```python
from build123d import *

# Parameters (mm, degrees)
ESQUISSE1_W             = 148.59
ESQUISSE1_H             = 2.5
ESQUISSE1_H_2           = 20
BOSS_EXTRU_2_DEPTH      = 5
BOSS_EXTRU_4_DEPTH      = 0.001
BOSS_EXTRU_4_DEPTH_BACK = 2.5
ESQUISSE2_W             = 148.59
ESQUISSE2_H             = 43.5
ESQUISSE3_R             = 2
ENL_V_MAT_EXTRU_1_DEPTH = 5
BOSS_EXTRU_9_DEPTH      = 148
ENL_V_MAT_EXTRU_2_DEPTH = 148
ENL_V_MAT_EXTRU_3_DEPTH = 158
ESQUISSE7_W             = 74.295
ESQUISSE7_H             = 5.75
BOSS_EXTRU_10_DEPTH     = 11
ESQUISSE8_W             = 148
ESQUISSE8_H             = 6.4
BOSS_EXTRU_11_DEPTH     = 40


with BuildPart() as part:
    # Esquisse1 → Boss.-Extru.2 (new body)
    with BuildSketch(Plane(origin=(0, 0, 0), x_dir=(1, 0, 0), z_dir=(0, 1, 0))):
        with Locations((-5.161134174, 17.745562161)):
            Rectangle(ESQUISSE1_W, ESQUISSE1_H)
        with Locations((-5.161134174, 28.995562161)):
            Rectangle(ESQUISSE1_W, ESQUISSE1_H_2)
    extrude(amount=BOSS_EXTRU_2_DEPTH)

    # Esquisse2 → Boss.-Extru.4 (add, two sides: drawn at the far end of the back side and taken through both)
    with BuildSketch(Plane(origin=(0, 0, -38.995562161), x_dir=(-1, 0, 0), z_dir=(0, 0, -1)).offset(-BOSS_EXTRU_4_DEPTH_BACK)):
        with Locations((5.161134174, 26.75)):
            Rectangle(ESQUISSE2_W, ESQUISSE2_H)
    extrude(amount=BOSS_EXTRU_4_DEPTH + BOSS_EXTRU_4_DEPTH_BACK)

    # Esquisse3 → Enlèv. mat.-Extru.1 (cut)
    with BuildSketch(Plane.XZ):
        with Locations(Location((-69.456134174, -25.995562161, 0), (0, 0, 270))):
            Circle(ESQUISSE3_R)
        with Locations(Location((59.133865826, -25.995562161, 0), (0, 0, 270))):
            Circle(ESQUISSE3_R)
    extrude(amount=-ENL_V_MAT_EXTRU_1_DEPTH, mode=Mode.SUBTRACT)

    # Esquisse4 → Boss.-Extru.9 (add)
    with BuildSketch(Plane.ZY.offset(79.456134174)):
        Polygon((-38.996562161, 5), (-38.996562161, 48.5), (-53.996562161, 48.5), (-53.996562161, 20), align=None)
    extrude(amount=-BOSS_EXTRU_9_DEPTH)

    # Esquisse5 → Enlèv. mat.-Extru.2 (cut)
    with BuildSketch(Plane.XY.offset(-36.495562161)):
        with BuildLine():
            ThreePointArc((31.986365826, 33.75), (28.486365826, 30.25), (31.986365826, 26.75))
            Line((31.986365826, 26.75), (31.986365826, 33.75))
        make_face()
        with BuildLine():
            Line((31.986365826, 33.75), (31.986365826, 26.75))
            ThreePointArc((31.986365826, 26.75), (34.46123956, 27.775126266), (35.486365826, 30.25))
            ThreePointArc((35.486365826, 30.25), (34.46123956, 32.724873734), (31.986365826, 33.75))
        make_face()
        with BuildLine():
            ThreePointArc((-38.808634174, 30.25), (-39.83376044, 32.724873734), (-42.308634174, 33.75))
            Line((-42.308634174, 33.75), (-42.308634174, 26.75))
            ThreePointArc((-42.308634174, 26.75), (-39.83376044, 27.775126266), (-38.808634174, 30.25))
        make_face()
        with BuildLine():
            Line((-42.308634174, 26.75), (-42.308634174, 33.75))
            ThreePointArc((-42.308634174, 33.75), (-45.808634174, 30.25), (-42.308634174, 26.75))
        make_face()
    extrude(amount=-ENL_V_MAT_EXTRU_2_DEPTH, mode=Mode.SUBTRACT)

    # Esquisse6 → Enlèv. mat.-Extru.3 (cut)
    with BuildSketch(Plane(origin=(68.543865826, 0, 0), x_dir=(0, 0, -1), z_dir=(1, 0, 0))):
        Polygon((38.996562161, 43.015232444), (49.10993279, 43.015232444), (49.10993279, 20.45031737), (38.996562161, 10.336946741), align=None)
    extrude(amount=-ENL_V_MAT_EXTRU_3_DEPTH, mode=Mode.SUBTRACT)

    # Esquisse7 → Boss.-Extru.10 (add)
    with BuildSketch(Plane.XY.offset(-36.495562161)):
        with Locations((-5.161134174, 45.625)):
            Rectangle(ESQUISSE7_W, ESQUISSE7_H)
    extrude(amount=BOSS_EXTRU_10_DEPTH)

    # Esquisse8 → Boss.-Extru.11 (add)
    with BuildSketch(Plane(origin=(0, 48.5, 0), x_dir=(1, 0, 0), z_dir=(0, 1, 0))):
        with Locations((-5.456134174, 50.796562161)):
            Rectangle(ESQUISSE8_W, ESQUISSE8_H)
    extrude(amount=BOSS_EXTRU_11_DEPTH)


solid = part.part
```
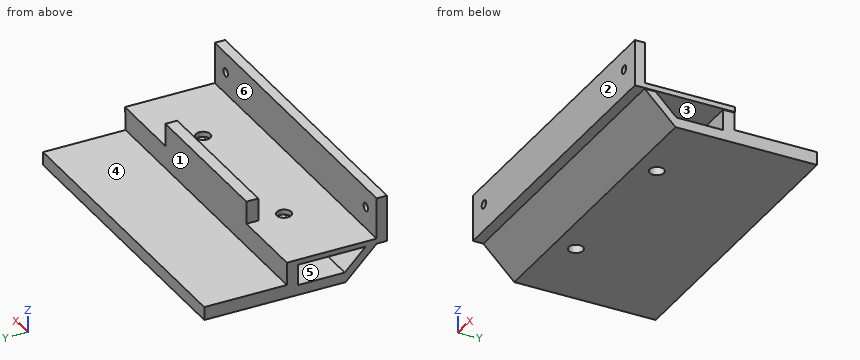
Model file for the job. Use its own axes, mm. Face numbers are marked on the shaded views. A direction names the side the tool comes from. Coordinates: 2 decimals unless noted, no trailing zeros. Loops run counter-clockwise (first coordinate to the right, second up) from the corner with the lowest first, then second, coordinate; pieces in that order, holes last. Notation, with made-up numbers: (-29.75, -0.5) - (-17.75, -0.5) arc R29 cw to (-17.75, 24.5) - close; hole circle Ø10 at (-31.5, -8). An arc over 180 degrees is marked (long way). Answer as a JSON object with one key per item and string values. Group by question number.
(1) Flat gauge pins, fed straight in: pin 1 (3 mm diameter, centred on x = -26.5, z = -43, fed in from -Y); pin 2 (1.5 mm diameter, centred on x = -63.5, y = 34.5, fed in from +Z); pin 3 (1.7 mm diameter, centred on x = -6.5, y = 46, fed in from +Z). Where does each tip first touch, or does it go through?
(2) Cut at D-D (y = 70.5). Give the cut face in (x, z).
(3) Two-plate mould, pull along Y, no slides. Class the marked faces 1, 2 and 3: released by +Y, released by -Y, zero draft, split by the parting line, or undercut.
(4) Cut at C-C (y = 7). Give the cut face in (x, z).
(5) Cut at A-A (y = 40). Give the cut face in (x, z), then the cut area to 3 significant figures.
(6) Tool access for the marked faces 4, 5 and 6: list every direction of +Z, -Z, +X, -X, +Y, -Y with a clear straight run to the whole face (end or side of a thin tool).
(7) Probe line 1 along X through (y, z) = (4, -25); line 2 along Z through (x, y) = (28.5, 34.5); line 3 along Y through (x, z) = (-2, -26). List the from-to ranges inside material, lowest first.
Geometry says:
{
 "1": {"pin 1": "stops at y = 7.5", "pin 2": "stops at z = -36.5", "pin 3": "stops at z = -25.5"},
 "2": {"outline": "(-79.46, -54) - (68.54, -54) - (68.54, -47.6) - (-79.46, -47.6) - close"},
 "3": {"face 1": "released by +Y", "face 2": "released by -Y", "face 3": "undercut"},
 "4": {"outline": "(-79.46, -41) - (68.54, -41) - (68.54, -39) - (69.13, -39) - (69.13, -36.5) - (-79.46, -36.5) - close"},
 "5": {"outline": "(-79.46, -54) - (68.54, -54) - (68.54, -49.11) - (-79.46, -49.11) - close; (-79.46, -39) - (69.13, -39) - (69.13, -36.5) - (-79.46, -36.5) - close", "area": "1,090 mm^2"},
 "6": {"face 4": "+Z, +X, -X, +Y", "face 5": "+X, -X", "face 6": "+Z, +X, -X"},
 "7": {"line 1": "x = -79.46 to -71.19, -67.72 to 57.4, 60.87 to 69.13", "line 2": "z = -54 to -49.11, -39 to -36.5", "line 3": "y = 0 to 5, 42.75 to 48.5"}
}
